```python
from build123d import *

# Parameters (mm, degrees)
F0_R     = 6
F1_DEPTH = 10
F2_W     = 40
F2_H     = 52
F3_DEPTH = 10
F4_R     = 11.99999
F5_R     = 8
F7_DEPTH = 102.001


# Not quite as in the source:
# - a fillet or chamfer is up to 0.001 mm smaller than in the source, because OpenCascade refuses the exact size


with BuildPart() as f1:
    # F0 (on Front) → F1 (new body)
    with BuildSketch(Plane.XZ):
        with BuildLine():
            Line((32, 52), (0, 52))
            Line((0, 52), (0, 0))
            Line((0, 0), (32, 0))
            Line((32, 0), (32, 12))
            Line((32, 12), (88, 12))
            ThreePointArc((88, 12), (102, 26), (88, 40))
            Line((88, 40), (32, 40))
            Line((32, 40), (32, 52))
        make_face()
        with Locations((20, 12)):
            Circle(F0_R, mode=Mode.SUBTRACT)
        with Locations((20, 40)):
            Circle(F0_R, mode=Mode.SUBTRACT)
        with BuildLine():
            ThreePointArc((44, 20), (38, 26), (44, 32))
            Line((44, 32), (88, 32))
            ThreePointArc((88, 32), (94, 26), (88, 20))
            Line((88, 20), (44, 20))
        make_face(mode=Mode.SUBTRACT)
    extrude(amount=F1_DEPTH)

    # F2 (on Right) → F3 (join)
    with BuildSketch(Plane.YZ):
        with Locations((-20, 26)):
            Rectangle(F2_W, F2_H)
    extrude(amount=F3_DEPTH)

    # F4 (radius 12 in the source; OpenCascade refuses exactly that, so slightly less here)
    f4_edges = [f1.edges().sort_by_distance(p)[0] for p in [
        (32, -5, 40),
        (32, -5, 12),
    ]]
    fillet(f4_edges, radius=F4_R)

    # F5
    f5_edges = [f1.edges().sort_by_distance(p)[0] for p in [
        (5, -40, 0),
        (5, -40, 52),
    ]]
    fillet(f5_edges, radius=F5_R)

    # F6 (on Right) → F7 (cut, through all)
    with BuildSketch(Plane.YZ):
        with BuildLine():
            Line((-24, 11), (-32, 11))
            ThreePointArc((-32, 11), (-35, 8), (-32, 5))
            Line((-32, 5), (-24, 5))
            ThreePointArc((-24, 5), (-21, 8), (-24, 11))
        make_face()
    extrude(amount=F7_DEPTH, mode=Mode.SUBTRACT)

    # F9: F1 across plane


with BuildPart() as f1_1:
    add(f1.part)
    add(f1.part.mirror(Plane(origin=(11.5185185185, -11.5185185185, 26), x_dir=(1, 0, 0), z_dir=(0, 0, 1))), mode=Mode.INTERSECT)


solid = f1_1.part
```
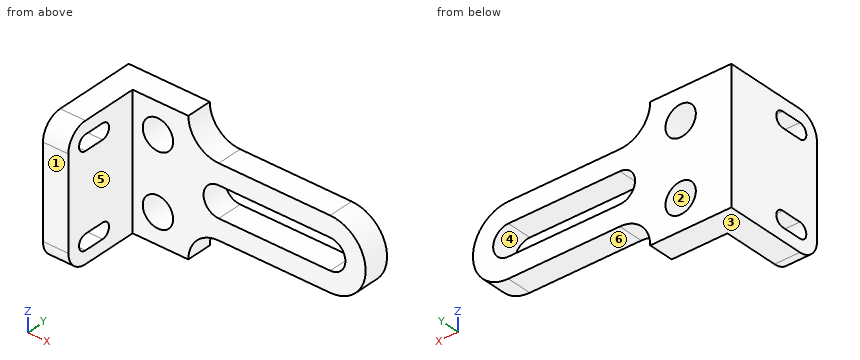
Model file for the job. Use its own axes, mm. Face numbers are marked on the shaded views. A direction names the side the tool comes from. Coordinates: 2 decimals unless noted, no trailing zeros. Write each loop counter-clockwise with the first axis right and the second up, starting at its lowest first coordinate (ties: lowest second). Pieces come first, ordered by that corner, then holes. Notation, with made-up numbers: (27.5, 55.5) - (59.5, 55.5) arc R22 cw to (59.5, 74.5) - close; hole circle Ø2 at (8, 10). An arc over 180 degrees is marked (long way). One line per question, with ' | ' between items. Start each with the question number.
Q1. Cut at D-D, the plane y = -36.5. List the corners of the cut face in (x, z), then the cut area to 3 significant figures.
Q2. Cut at A-A, the plane x = 62.5. List the corners of the cut face in (y, z).
Q3. Pull direction Z, two halves, no side cores. Call the marked faces 1, 2 and 3: pulls with the +Z half, pulls with the -Z half, needs draft (parallel to the pull), parting line crosses it, or undercut.
Q4. Pin check, flat tips, straight feed: pin 1 (11 mm diameter, centred on x = 64, y = -7, fed in from -Z); pin 2 (3 mm diameter, centred on x = 76, y = -3.5, fed in from +Z); pin 3 (15.5 mm diameter, centred on x = 39.5, z = 13.5, fed in from -Y). Stop position of each tip, or through.
Q5. Cut at C-C, the plane z = 7. List the corners of the cut face in (x, y), then the cut area to 3 significant figures.
Q6. 3-axis set-ups, long thin cutter, end or side, ignore diameter. For the marked faces 4, 5 and 6: which of +Z, -Z, +X, -X, +Y, -Y reach the whole face in a straight line?
Q7. Cut at B-B, the plane z = 26. List the corners of the cut face in (x, y), then the cut area to 3 significant figures.
Q8. Drill centre lines: line 1 (Z direction, x = 20, y = -2.25); line 2 (Z direction, x = 63, y = -8.5); line 3 (Y direction, x = 27, z = 12.5). Where is each one in solid material? Low to high. Write a range as [from, to].
Answer below:
1) outline: (0, 1.39) - (10, 1.39) - (10, 50.61) - (0, 50.61) - close | area: 492 mm^2
2) outline: (-10, 12) - (0, 12) - (0, 20) - (-10, 20) - close; (-10, 32) - (0, 32) - (0, 40) - (-10, 40) - close
3) face 1: needs draft | face 2: undercut | face 3: pulls with the -Z half
4) pin 1: z = 12 | pin 2: z = 40 | pin 3: y = -10
5) outline: (0, -39.94) - (10, -39.94) - (10, -34.83) - (0, -34.83) - close; (0, -21.17) - (10, -21.17) - (10, -10) - (16.68, -10) - (16.68, 0) - (0, 0) - close; (23.32, -10) - (34.25, -10) - (34.25, 0) - (23.32, 0) - close | area: 439 mm^2
6) face 4: +Y, -Y | face 5: +Z, -Z, +X, -Y | face 6: -Z, +X, +Y, -Y
7) outline: (0, -40) - (10, -40) - (10, -10) - (38, -10) - (38, 0) - (0, 0) - close; (94, -10) - (102, -10) - (102, 0) - (94, 0) - close | area: 760 mm^2
8) line 1: [0, 6], [18, 34], [46, 52] | line 2: [12, 20], [32, 40] | line 3: [-10, 0]
